Autodesk Inventor part; units mm, degrees
ref_plane "YZ Plane" through (0, 0, 0) normal (1, 0, 0) x (0, 1, 0)
ref_plane "XZ Plane" through (0, 0, 0) normal (0, 1, 0) x (-1, 0, 0)
ref_plane "XY Plane" through (0, 0, 0) normal (0, 0, 1) x (1, 0, 0)
sketch "Sketch1" plane through (0, 0, 0) normal (0, 0, 1) x (1, 0, 0)
  line L0 (-7.3323, 0) -> (-3.6662, 6.35)
  line L1 (-3.6662, 6.35) -> (3.6662, 6.35)
  line L2 (3.6662, 6.35) -> (7.3323, 0)
  line L3 (7.3323, 0) -> (3.6662, -6.35)
  line L4 (3.6662, -6.35) -> (-3.6662, -6.35)
  line L5 (-3.6662, -6.35) -> (-7.3323, 0)
  circle A0 centre (0, 0) radius 1.5923 construction
  dimension "d0" = 12.7
extrude "Extrusion1" add sketch "Sketch1" along normal mid plane 53.975
sketch "Sketch2" plane through (0, 0, 26.9875) normal (0, 0, 1) x (1, 0, 0)
  line L0 (3.6662, 6.35) -> (-3.6662, 6.35)
  line L1 (-3.6662, -6.35) -> (3.6662, -6.35)
  line L2 (3.6662, -6.35) -> (7.3323, 0)
  line L3 (7.3323, 0) -> (3.6662, 6.35)
  line L4 (3.6662, 6.35) -> (-3.6662, 6.35)
  line L5 (-3.6662, 6.35) -> (-7.3323, 0)
  line L6 (-7.3323, 0) -> (-3.6662, -6.35)
  circle A0 centre (0, 0) radius 7.62
  line L7 (1.5, -2.5) -> (-1.5, -2.5)
  line L8 (-1.5, -2.5) -> (-1.5, 2.5)
  line L9 (-1.5, 2.5) -> (1.5, 2.5)
  line L10 (1.5, 2.5) -> (1.5, -2.5)
  line L11 (1.5, -2.5) -> (-1.5, 2.5) construction
  line L12 (-1.5, -2.5) -> (1.5, 2.5) construction
  dimension "d5" = 15.24
  dimension "d6" = 3
  dimension "d7" = 5
extrude "Extrusion2" add sketch "Sketch2" along normal blind 9.525 contours L3 L2 L1 L6 L5 L0 | A0
sketch "Sketch3" plane through (0, 0, -26.9875) normal (0, 0, -1) x (-1, 0, 0)
  line L0 (2.54, -2.54) -> (-2.54, -2.54)
  line L1 (-2.54, -2.54) -> (-2.54, 2.54)
  line L2 (-2.54, 2.54) -> (2.54, 2.54)
  line L3 (2.54, 2.54) -> (2.54, -2.54)
  line L4 (2.54, -2.54) -> (-2.54, 2.54) construction
  line L5 (-2.54, -2.54) -> (2.54, 2.54) construction
  point P0 (0, 0)
  dimension "d11" = 5.08
  dimension "d12" = 5.08
extrude "Extrusion3" cut sketch "Sketch3" against normal blind 3.175
fillet "Fillet1" radius 0.381 4 edges at (2.54, 0, -26.9875) (0, 2.54, -26.9875) (0, -2.54, -26.9875) (-2.54, 0, -26.9875)
properties part number "Shaft"
Can you work these out from the model? Positions are in its coordinate system, mm. A direction names the side the tool comes from. Coordinates: 2 decimals unless noted, no trailing zeros. Write each loop counter-clockwise with the first axis right and the second up, starting at its lowest first coordinate (ties: lowest second). Pieces come first, ordered by that corner, then holes. Notation, with made-up numbers: M -1.75,-4 L 34.25,-4 A20 cw 34.25,28 Z; hole C 44,76.5 d3. An arc over 180 degrees is marked long. Write item = value, one per line. Start each with the question number.
Q1. I'm going to push flat-ended pins straight in: pin 1 (2.5 mm diameter, centred on x = 0.5, y = 0, fed in from -Z); pin 2 (4 mm diameter, centred on x = -4, z = 28.5, fed in from +Y); pin 3 (3.5 mm diameter, centred on x = 1, z = -11.5, fed in from +Y). Where does each tip first touch, or does it pass through?
Q2. If we section it at A-A, the plane z = 31.5: Write out the boundary of the cut face in (x, y), then the cut area to 3 significant figures.
Q3. If we section it at B-B, the plane x = 0: Write out the boundary of the cut face in (y, z).
Q4. If we section it at D-D, the plane y = 4.75: Write out the boundary of the cut face in (x, z).
Q5. If I drill on L1, parallel to Z at x = -1, y = -0.5; L2, parallel to Z at x = 5.75, y = 3; L3, parallel to Y at x = -0.75, z = 11.5, over which ranges is the centre line in solid material (lowest first)? Write a range as [from, to].
Q6. Thinking about a two-plate mould opening in Y: for faces 5 (the face through (0, 2.5, 32)), 6 (the face through (6, -3, 26.988)), 7 (the face through (-5.474, -3.219, -0.378)), 8 (the face through (5.474, 3.219, -0.378)), which applies, released by +Y, released by -Y, zero draft, split by the parting line, or undercut?
Q7. On a 3-axis mill with a long thin cutter (end or side, diameter ignored), from which of +Z, -Z, +X, -X, +Y, -Y can I reach the whole of each face in a straight line? I mean faces 1 (the face through (2.54, 0, -25)), 2 (the face through (-5.525, 3.131, -0.378)), 3 (the face through (0, 0, 26.988)), 4 (the face through (0, 6.35, 0)). Say none if no direction works.
Q8. If we section it at C-C, the plane z = 13.5: Write out the boundary of the cut face in (x, y).
Check sheet entries:
q1.pin_1 = -23.81
q1.pin_2 = 7.35
q1.pin_3 = 6.35
q2.outline = C 0,0 d15.24; hole M -1.5,-2.5 L 1.5,-2.5 L 1.5,2.5 L -1.5,2.5 Z
q2.area = 167 mm²
q3.outline = M -7.62,26.99 L -6.35,26.99 L -6.35,-26.99 L -2.92,-26.99 A0.38 ccw -2.54,-26.61 L -2.54,-23.81 L 2.54,-23.81 L 2.54,-26.61 A0.38 ccw 2.92,-26.99 L 6.35,-26.99 L 6.35,26.99 L 7.62,26.99 L 7.62,36.51 L 2.5,36.51 L 2.5,26.99 L -2.5,26.99 L -2.5,36.51 L -7.62,36.51 Z
q4.outline = M -5.96,26.99 L -4.59,26.99 L -4.59,-26.99 L 4.59,-26.99 L 4.59,26.99 L 5.96,26.99 L 5.96,36.51 L -5.96,36.51 Z
q5.L1 = [-23.81, 26.99]
q5.L2 = [26.99, 36.51]
q5.L3 = [-6.35, 6.35]
q6.face_5 = undercut
q6.face_6 = zero draft
q6.face_7 = released by -Y
q6.face_8 = released by +Y
q7.face_1 = -Z
q7.face_2 = -Z, -X, +Y
q7.face_3 = +Z
q7.face_4 = -Z, +X, -X, +Y
q8.outline = M -7.33,0 L -3.67,-6.35 L 3.67,-6.35 L 7.33,0 L 3.67,6.35 L -3.67,6.35 Z
